from build123d import *

# Parameters (mm, degrees)
SKETCH_1_W                  = 320
SKETCH_1_H                  = 200
SM_BASE_FLANGE_1_DEPTH      = 4
HOLE_WIZARD_1_AT_2_COUNT    = 2
HOLE_WIZARD_1_AT_2_PITCH    = 30
HOLE_WIZARD_1_AT_3_COUNT    = 2
HOLE_WIZARD_1_AT_3_PITCH    = 43.863424399
HOLE_WIZARD_1_AT_4_COUNT    = 2
HOLE_WIZARD_1_AT_4_PITCH    = 32
HOLE_WIZARD_1_AT_5_COUNT    = 2
HOLE_WIZARD_1_AT_5_PITCH    = 129.031004026
HOLE_WIZARD_1_AT_6_COUNT    = 2
HOLE_WIZARD_1_AT_6_PITCH    = 125
HOLE_WIZARD_1_AT_7_COUNT    = 2
HOLE_WIZARD_1_AT_7_PITCH    = 158.268758762
HOLE_WIZARD_1_AT_8_COUNT    = 2
HOLE_WIZARD_1_AT_8_PITCH    = 155
SKETCH_9_W                  = 30
SKETCH_9_H                  = 45
SM_BASE_FLANGE_1_2_DEPTH    = 4
SKETCH_27_W                 = 123
SKETCH_27_H                 = 5
CUT_EXTRUDE_2_DEPTH         = 10
SM_EDGE_FLANGE_1_DEPTH      = 100
SM_EDGE_FLANGE_1_BEND_DEPTH = 100
HOLE_START                  = -108.5
HOLE_WIZARD_8_2_8_2_1_DEPTH = 217
F_5_2_5_2_DIAMETER_HOLE1_D  = 5.2
CUT_EXTRUDE_1_REACH         = 223.199
SKETCH_21_W                 = 30
SKETCH_21_H                 = 30
HOLE_WIZARD_M3_2_D          = 2.5
OTHER_START                 = -108.5
OTHER_1_DEPTH               = 217
OTHER_START_2               = -4
OTHER_2_DEPTH               = 4
OTHER_2_2_DEPTH             = 4
HOLE_WIZARD_M3_1_D          = 2.5
HOLE_WIZARD_M3_3_D          = 2.5


# Read off the part's stored shape, not the designer's step: Ø8.2 (8.2) 直径槽口1, 断开-边角1, 断开-边角2
# Sheet-metal steps are written as plain solids
with BuildPart() as part:
    # Sketch 1 → Sm Base Flange 1 (new body)
    with BuildSketch(Plane(origin=(0, 0, 0), x_dir=(1, 0, 0), z_dir=(0, 1, 0))):
        Rectangle(SKETCH_1_W, SKETCH_1_H)
    extrude(amount=-SM_BASE_FLANGE_1_DEPTH)

    # 草图7 → 打孔尺寸开槽半沉头螺钉的类型1 (revolve, cut)
    with BuildSketch(Plane(origin=(-154, 0, 62.5), x_dir=(0, 0, 1), z_dir=(1, 0, 0))):
        Polygon((0, 0), (0, 4), (2.75, 4), (2.75, 2.55), (5.3, 0), align=None)
    hole_wizard_1 = revolve(axis=Axis((-154, 6.35, 62.5), (0, -1, 0)), mode=Mode.SUBTRACT)

    # 打孔尺寸开槽半沉头螺钉的类型1 at 2: 打孔尺寸开槽半沉头螺钉的类型1 ×2
    with Locations(*[(0, 0, i * HOLE_WIZARD_1_AT_2_PITCH) for i in range(1, HOLE_WIZARD_1_AT_2_COUNT)]):
        add(hole_wizard_1, mode=Mode.SUBTRACT)

    # 打孔尺寸开槽半沉头螺钉的类型1 at 3: 打孔尺寸开槽半沉头螺钉的类型1 ×2
    with Locations(*[Vector(0.7295372041400852, 0, 0.6839411288813297) * (i * HOLE_WIZARD_1_AT_3_PITCH) for i in range(1, HOLE_WIZARD_1_AT_3_COUNT)]):
        add(hole_wizard_1, mode=Mode.SUBTRACT)

    # 打孔尺寸开槽半沉头螺钉的类型1 at 4: 打孔尺寸开槽半沉头螺钉的类型1 ×2
    with Locations(*[(i * HOLE_WIZARD_1_AT_4_PITCH, 0, 0) for i in range(1, HOLE_WIZARD_1_AT_4_COUNT)]):
        add(hole_wizard_1, mode=Mode.SUBTRACT)

    # 打孔尺寸开槽半沉头螺钉的类型1 at 5: 打孔尺寸开槽半沉头螺钉的类型1 ×2
    with Locations(*[Vector(0.24800241028513723, 0, -0.9687594151763185) * (i * HOLE_WIZARD_1_AT_5_PITCH) for i in range(1, HOLE_WIZARD_1_AT_5_COUNT)]):
        add(hole_wizard_1, mode=Mode.SUBTRACT)

    # 打孔尺寸开槽半沉头螺钉的类型1 at 6: 打孔尺寸开槽半沉头螺钉的类型1 ×2
    with Locations(*[(0, 0, -i * HOLE_WIZARD_1_AT_6_PITCH) for i in range(1, HOLE_WIZARD_1_AT_6_COUNT)]):
        add(hole_wizard_1, mode=Mode.SUBTRACT)

    # 打孔尺寸开槽半沉头螺钉的类型1 at 7: 打孔尺寸开槽半沉头螺钉的类型1 ×2
    with Locations(*[Vector(0.20218772327747656, 0, -0.979346784625278) * (i * HOLE_WIZARD_1_AT_7_PITCH) for i in range(1, HOLE_WIZARD_1_AT_7_COUNT)]):
        add(hole_wizard_1, mode=Mode.SUBTRACT)

    # 打孔尺寸开槽半沉头螺钉的类型1 at 8: 打孔尺寸开槽半沉头螺钉的类型1 ×2
    with Locations(*[(0, 0, -i * HOLE_WIZARD_1_AT_8_PITCH) for i in range(1, HOLE_WIZARD_1_AT_8_COUNT)]):
        add(hole_wizard_1, mode=Mode.SUBTRACT)

    # 草图9 → Sm Base Flange 1 2 (add)
    with BuildSketch(Plane(origin=(0, 0, 0), x_dir=(1, 0, 0), z_dir=(0, 1, 0))):
        with Locations((-78, -122.5)):
            Rectangle(SKETCH_9_W, SKETCH_9_H)
    extrude(amount=-SM_BASE_FLANGE_1_2_DEPTH)

    # 草图27 → 切除-拉伸2 (cut)
    with BuildSketch(Plane(origin=(0, 0, 0), x_dir=(1, 0, 0), z_dir=(0, 1, 0))):
        with Locations((-1.5, -97.5)):
            Rectangle(SKETCH_27_W, SKETCH_27_H)
        with Locations((-1.5, 97.5)):
            Rectangle(SKETCH_27_W, SKETCH_27_H)
    extrude(amount=-CUT_EXTRUDE_2_DEPTH, mode=Mode.SUBTRACT)

    # 边线-法兰1 section (across the edge) → 边线-法兰1 (add)
    with BuildSketch(Plane(origin=(60, 0, 104.5), x_dir=(0, 0, -1), z_dir=(1, 0, 0))):
        with BuildLine():
            Line((-4, 0.5), (-4, 48))
            Line((-4, 48), (0, 48))
            Line((0, 48), (0, 0.5))
            ThreePointArc((0, 0.5), (0.146446609, 0.146446609), (0.5, 0))
            Line((0.5, 0), (4.5, 0))
            Line((4.5, 0), (4.5, -4))
            Line((4.5, -4), (0.5, -4))
            ThreePointArc((0.5, -4), (-2.681980515, -2.681980515), (-4, 0.5))
        make_face()
    extrude(amount=SM_EDGE_FLANGE_1_DEPTH)

    # 边线-法兰1 section 2 (across the edge) → 边线-法兰1 bend (add)
    with BuildSketch(Plane(origin=(160, 0, -104.5), x_dir=(0, 0, 1), z_dir=(-1, 0, 0))):
        with BuildLine():
            Line((-4, 0.5), (-4, 48))
            Line((-4, 48), (0, 48))
            Line((0, 48), (0, 0.5))
            ThreePointArc((0, 0.5), (0.146446609, 0.146446609), (0.5, 0))
            Line((0.5, 0), (4.5, 0))
            Line((4.5, 0), (4.5, -4))
            Line((4.5, -4), (0.5, -4))
            ThreePointArc((0.5, -4), (-2.681980515, -2.681980515), (-4, 0.5))
        make_face()
    extrude(amount=SM_EDGE_FLANGE_1_BEND_DEPTH)

    # Ø8.2 (8.2) 直径槽口1 outline → Ø8.2 (8.2) 直径槽口1 (cut)
    with BuildSketch(Plane.XY.offset(HOLE_START)):
        with BuildLine():
            ThreePointArc((145.9, 24.6), (150, 20.5), (154.1, 24.6))
            Line((154.1, 24.6), (154.1, 36.4))
            ThreePointArc((154.1, 36.4), (150, 40.5), (145.9, 36.4))
            Line((145.9, 36.4), (145.9, 24.6))
        make_face()
        with BuildLine():
            ThreePointArc((65.9, 24.6), (70, 20.5), (74.1, 24.6))
            Line((74.1, 24.6), (74.1, 36.4))
            ThreePointArc((74.1, 36.4), (70, 40.5), (65.9, 36.4))
            Line((65.9, 36.4), (65.9, 24.6))
        make_face()
    extrude(amount=HOLE_WIZARD_8_2_8_2_1_DEPTH, mode=Mode.SUBTRACT)

    # Ø5.2 (5.2) Diameter Hole1 (through all)
    with Locations(Plane(origin=(0, 0, 0), x_dir=(1, 0, 0), z_dir=(0, 1, 0))):
        with Locations((-78, -137.5), (-78, -117.5)):
            Hole(F_5_2_5_2_DIAMETER_HOLE1_D / 2)

    # 草图21 → 切除-拉伸1 (cut, up to next)
    with BuildSketch(Plane(origin=(0, 0, 0), x_dir=(1, 0, 0), z_dir=(0, 1, 0)), mode=Mode.PRIVATE) as cut_extrude_1_sk1:
        with Locations((-85, 0)):
            Rectangle(SKETCH_21_W, SKETCH_21_H)
    cut_extrude_1_tool1 = extrude(cut_extrude_1_sk1.sketch, amount=-CUT_EXTRUDE_1_REACH, mode=Mode.PRIVATE) & part.part
    add(cut_extrude_1_tool1.solids().sort_by_distance((-85, 0, 0))[0], mode=Mode.SUBTRACT)

    # M3 螺纹孔2 (through all)
    with Locations(Plane(origin=(0, 0, 0), x_dir=(1, 0, 0), z_dir=(0, 1, 0))):
        with Locations((-106, 6), (-106, -6)):
            Hole(HOLE_WIZARD_M3_2_D / 2)

    # Other 1 outline → Other 1 (cut)
    with BuildSketch(Plane.XY.offset(OTHER_START)):
        with BuildLine():
            ThreePointArc((60, 43), (61.464466094, 46.535533906), (65, 48))
            Line((65, 48), (60, 48))
            Line((60, 48), (60, 43))
        make_face()
        with BuildLine():
            ThreePointArc((155, 48), (158.535533906, 46.535533906), (160, 43))
            Line((160, 43), (160, 48))
            Line((160, 48), (155, 48))
        make_face()
    extrude(amount=OTHER_1_DEPTH, mode=Mode.SUBTRACT)

    # Other 2 outline → Other 2 (cut)
    with BuildSketch(Plane(origin=(0, 0, 0), x_dir=(1, 0, 0), z_dir=(0, 1, 0)).offset(OTHER_START_2)):
        with BuildLine():
            ThreePointArc((-63, -140), (-64.464466094, -143.535533906), (-68, -145))
            Line((-68, -145), (-63, -145))
            Line((-63, -145), (-63, -140))
        make_face()
        with BuildLine():
            ThreePointArc((-88, -145), (-91.535533906, -143.535533906), (-93, -140))
            Line((-93, -140), (-93, -145))
            Line((-93, -145), (-88, -145))
        make_face()
        with BuildLine():
            ThreePointArc((-155, -100), (-158.535533906, -98.535533906), (-160, -95))
            Line((-160, -95), (-160, -100))
            Line((-160, -100), (-155, -100))
        make_face()
        with BuildLine():
            ThreePointArc((-160, 95), (-158.535533906, 98.535533906), (-155, 100))
            Line((-155, 100), (-160, 100))
            Line((-160, 100), (-160, 95))
        make_face()
    extrude(amount=OTHER_2_DEPTH, mode=Mode.SUBTRACT)

    # Other 2 2 outline → Other 2 2 (add)
    with BuildSketch(Plane(origin=(0, 0, 0), x_dir=(1, 0, 0), z_dir=(0, 1, 0)).offset(OTHER_START_2)):
        with BuildLine():
            ThreePointArc((-58, 95), (-61.535533906, 96.464466094), (-63, 100))
            Line((-63, 100), (-63, 95))
            Line((-63, 95), (-58, 95))
        make_face()
        with BuildLine():
            Line((-63, -95), (-63, -100))
            ThreePointArc((-63, -100), (-61.535533906, -96.464466094), (-58, -95))
            Line((-58, -95), (-63, -95))
        make_face()
        with BuildLine():
            Line((-93, -100), (-98, -100))
            ThreePointArc((-98, -100), (-94.464466094, -101.464466094), (-93, -105))
            Line((-93, -105), (-93, -100))
        make_face()
    extrude(amount=OTHER_2_2_DEPTH)

    # M3 螺纹孔1 (through all)
    with Locations(Plane(origin=(0, 0, 0), x_dir=(1, 0, 0), z_dir=(0, 1, 0))):
        with Locations((-6, -88), (11, -88)):
            Hole(HOLE_WIZARD_M3_1_D / 2)

    # M3 螺纹孔3 (through all)
    with Locations(Plane(origin=(0, 0, 0), x_dir=(1, 0, 0), z_dir=(0, 1, 0))):
        with Locations((-88, -121.5), (-88, -133.5)):
            Hole(HOLE_WIZARD_M3_3_D / 2)


solid = part.part
Geometry check sheet. Reference: the model listing, model coordinates, mm. A direction names the side the tool comes from. Coordinates: 2 decimals unless noted, no trailing zeros. Order: outer loops, then holes, each group sorted by start corner. A loop starts at its lowest first (then second) coordinate and runs counter-clockwise, first axis right, second up. Notation, with made-up numbers: (16, 53.5) - (56, 53.5) arc R11 ccw to (56, 59.5) - close; hole circle Ø4 at (57.25, 30). An arc over 180 degrees is marked (long way). Answer in a Markdown table with one row per item. Add a question column.
1) Cross-section at B-B, the plane x = 123. Record the cut outline in (y, z), then the cut area to 3 significant figures.
2) Release check for a two-part mould opening along Z. For faces 3 (the flat face through (109, 24, 108.5)), 4 (the flat face through (60, 15, 105)), 5 (the conical face through (-156.885, -2.39, -62.879)), 6 (the flat face through (111, 25, -104.5)) record: +Z half, -Z half, draft (parallel to the pull), parting line (faces both ways), or undercut.
3) Gauge pin test, flat ends, axial feed: P1, Ø4.5, axis at x = -81, y = -1.5, coming from the -Z side; P2, Ø3.5, axis at x = -122, z = -92.5, coming from the +Y side; P3, Ø4.5, axis at y = 33, z = -107, coming from the -X side; P4, Ø3, axis at x = -6, z = 88, coming from the +Y side. Record the tip position at first contact, or that the pin passes through.
4) Cross-section at D-D, the plane z = 75. Record the cut outline in (x, y), then the cut area to 3 significant figures.
5) Set-up check for faces 1 (the flat face through (109, 25, 104.5)), 2 (the conical face through (-156.885, -2.39, 62.121)): record each of +Z, -Z, +X, -X, +Y, -Y from which the full face is reachable in a straight line by a thin tool's end or side.
6) Cross-section at C-C, the plane y = 32. Record the cut outline in (x, z).
7) Cross-section at A-A, the plane y = 12. Record the cut outline in (x, z), then the cut area to 3 significant figures.
8) Material ranges on line 1 along X through (y, z) = (-1.8, 88); line 2 along Z through (x, y) = (-154, -3.05); line 3 along X through (y, z) = (-2.8, 6), recorded low to high. Write a range as [from, to].
Check result:
| question | item | result |
|---|---|---|
| 1 | outline | (-4, -104) arc R4.5 ccw to (0.5, -108.5) - (48, -108.5) - (48, -104.5) - (0.5, -104.5) arc R0.5 cw to (0, -104) - (0, 104) arc R0.5 cw to (0.5, 104.5) - (48, 104.5) - (48, 108.5) - (0.5, 108.5) arc R4.5 ccw to (-4, 104) - close |
| 1 | area | 1,240 mm² |
| 2 | face 3 | +Z half |
| 2 | face 4 | draft |
| 2 | face 5 | undercut |
| 2 | face 6 | undercut |
| 3 | P1 | stops at z = -100 |
| 3 | P2 | passes through |
| 3 | P3 | stops at x = 60 |
| 3 | P4 | stops at y = 0 |
| 4 | outline | (-160, -4) - (160, -4) - (160, 0) - (-160, 0) - close |
| 4 | area | 1,280 mm² |
| 5 | face 1 | +X, -X, +Y |
| 5 | face 2 | +Y |
| 6 | outline | (60, -108.5) - (65.9, -108.5) - (65.9, -104.5) - (60, -104.5) - close; (60, 104.5) - (65.9, 104.5) - (65.9, 108.5) - (60, 108.5) - close; (74.1, -108.5) - (145.9, -108.5) - (145.9, -104.5) - (74.1, -104.5) - close; (74.1, 104.5) - (145.9, 104.5) - (145.9, 108.5) - (74.1, 108.5) - close; (154.1, -108.5) - (160, -108.5) - (160, -104.5) - (154.1, -104.5) - close; (154.1, 104.5) - (160, 104.5) - (160, 108.5) - (154.1, 108.5) - close |
| 7 | outline | (60, -108.5) - (160, -108.5) - (160, -104.5) - (60, -104.5) - close; (60, 104.5) - (160, 104.5) - (160, 108.5) - (60, 108.5) - close |
| 7 | area | 800 mm² |
| 8 | line 1 | x = [-160, -7.25], [-4.75, 9.75], [12.25, 160] |
| 8 | line 2 | z = [-100, -95.25], [-89.75, -65.25], [-59.75, 59.75], [65.25, 89.75], [95.25, 100] |
| 8 | line 3 | x = [-160, -107.25], [-104.75, -100], [-70, 160] |
